Input: part model. Units: mm. Frame: model coordinates. Face numbers are marked on the shaded views. A direction names the side the tool comes from. Coordinates: 2 decimals unless noted, no trailing zeros. Write each loop counter-clockwise with the first axis right and the second up, starting at its lowest first coordinate (ties: lowest second). Pieces come first, ordered by that corner, then holes. Notation, with made-up numbers: M 6,32 L 54,32 A17 ccw 54,54 Z; hole C -8.5,24.25 d7. An arc over 180 degrees is marked long. Write each question's results on one line, items separated by ' | '. Start each with the question number.
1. Section query A-A, the plane y = 2. Output: boundary loops of the cut face in (x, z), and give its area (3 significant figures).
2. First-contact query: pin 1 (2 mm diameter, centred on x = -19, y = 25, fed in from -Z); pin 2 (0.8 mm diameter, centred on y = 27.5, z = 2, fed in from +X); pin 3 (6 mm diameter, centred on x = -16.39, y = 20, fed in from -Z); pin 4 (2 mm diameter, centred on y = 27.5, z = 4.5, fed in from -X). Flat tips, straight axial feed; report the tip coordinate or a pass-through.
3. Section query C-C, the plane y = 20. Output: boundary loops of the cut face in (x, z), and give its area (3 significant figures).
4. Pull-direction query (X, two-part tool) for the marked faces 3, 4 and 5; classes: +X half, -X half, draft (parallel to the pull), parting line (faces both ways), or undercut.
5. Ray query, probe 1 along X at (y, z) = (14.5, 5.25); probe 2 along X at (y, z) = (0, 7.75); probe 3 along Y at (x, z) = (-16.5, 6.75). Return the intervals inside material, ascending.
6. Set-up query: the marked faces 1 and 2. Return all of +Z, -Z, +X, -X, +Y, -Y with unobstructed straight access to the full face (end or side cutting, diameter ignored); none if empty.
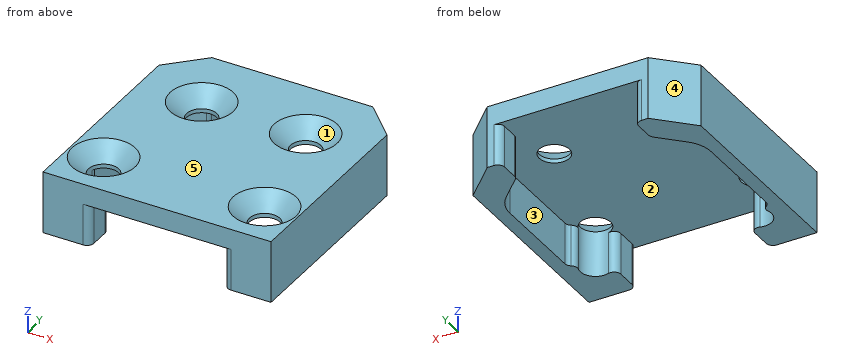
```python
from build123d import *

# Parameters (mm, degrees)
EXTRUDE1_DEPTH                                       = 9.25
CSK_FOR_M4_COUNTERSUNK_RAISED_HEAD_SCREW_D           = 4.5
CSK_FOR_M4_COUNTERSUNK_RAISED_HEAD_SCREW_CSINK_D     = 9.4
CSK_FOR_M4_COUNTERSUNK_RAISED_HEAD_SCREW_CSINK_ANGLE = 90
EXTRUDE2_DEPTH                                       = 6.2
FILLET1_R                                            = 1
FILLET2_R                                            = 1
FILLET3_R                                            = 5


with BuildPart() as part:
    # Sketch1 → Extrude1 (new body)
    with BuildSketch(Plane.XY):
        Polygon((3.357375606748374, 30), (-20.6426243932516, 30), (-25.642624393251616, 25.000000000000007), (-25.642624393251616, -4.999999999999999), (8.357375606748393, -4.999999999999999), (8.357375606748393, 25), align=None)
    extrude(amount=EXTRUDE1_DEPTH)

    # CSK for M4 Countersunk Raised Head Screw1 (through all)
    with Locations(Plane.XY.offset(9.249999999999995)):
        with Locations((-0.892624393, 20), (-16.392624393, 20), (-20.642624393, 2), (3.357375607, 2)):
            CounterSinkHole(CSK_FOR_M4_COUNTERSUNK_RAISED_HEAD_SCREW_D / 2, CSK_FOR_M4_COUNTERSUNK_RAISED_HEAD_SCREW_CSINK_D / 2, counter_sink_angle=CSK_FOR_M4_COUNTERSUNK_RAISED_HEAD_SCREW_CSINK_ANGLE)

    # Sketch6 → Extrude2 (cut)
    with BuildSketch(Plane(origin=(0, 0, 0), x_dir=(-1, 0, 0), z_dir=(0, 0, -1))):
        with BuildLine():
            Line((-1.357375606748385, -4.999999999999999), (-1.357375606748385, 1.9999999999999944))
            ThreePointArc((-1.357375606748385, 1.9999999999999944), (-1.9431620443752904, 3.4142135623730905), (-3.357375606748387, 3.9999999999999947))
            Line((-3.357375606748387, 3.9999999999999947), (-6.357375606748384, 3.9999999999999947))
            Line((-6.357375606748384, 3.9999999999999947), (-6.357375606748382, 20.999999999999996))
            Line((-6.357375606748382, 20.999999999999996), (-1.3573756067483855, 25.999999999999996))
            Line((-1.3573756067483855, 25.999999999999996), (-1.3573756067483855, 30))
            Line((-1.3573756067483855, 30), (18.642624393251616, 30))
            Line((18.642624393251616, 30), (18.642624393251616, 25.999999999999996))
            Line((18.642624393251616, 25.999999999999996), (23.642624393251612, 20.999999999999996))
            Line((23.642624393251612, 20.999999999999996), (23.642624393251612, 3.9999999999999947))
            Line((23.642624393251612, 3.9999999999999947), (20.642624393251616, 3.9999999999999947))
            ThreePointArc((20.642624393251616, 3.9999999999999947), (19.22841083087852, 3.4142135623730896), (18.642624393251616, 1.9999999999999944))
            Line((18.642624393251616, 1.9999999999999944), (18.642624393251616, -4.999999999999999))
            Line((18.642624393251616, -4.999999999999999), (-1.357375606748385, -4.999999999999999))
        make_face()
    extrude(amount=-EXTRUDE2_DEPTH, mode=Mode.SUBTRACT)

    # Fillet1
    # the kernel refuses this fillet: 1 mm, written as the material it takes off along each edge
    with BuildSketch(Plane(origin=(1.3573756067483842, -4.999999999999999, -2.5000000000000004), x_dir=(1, 0, 0), z_dir=(0, 0, 1))) as fillet1_piece_1:
        with BuildLine():
            CenterArc((FILLET1_R, FILLET1_R), FILLET1_R, 180, 90)
            Line((0, FILLET1_R), (0, 0))
            Line((0, 0), (FILLET1_R, 0))
        make_face()
    extrude(amount=8.700000000000001, mode=Mode.SUBTRACT)
    with BuildSketch(Plane(origin=(-18.642624393251616, -4.999999999999999, -2.5000000000000004), x_dir=(-1, 0, 0), z_dir=(0, 0, 1))) as fillet1_piece_2:
        with BuildLine():
            CenterArc((FILLET1_R, -FILLET1_R), FILLET1_R, 90, 90)
            Line((0, -FILLET1_R), (0, 0))
            Line((0, 0), (FILLET1_R, 0))
        make_face()
    extrude(amount=8.700000000000001, mode=Mode.SUBTRACT)
    with BuildSketch(Plane(origin=(-18.642624393251616, 30, -2.5000000000000004), x_dir=(-1, 0, 0), z_dir=(0, 0, 1))) as fillet1_piece_3:
        with BuildLine():
            CenterArc((FILLET1_R, FILLET1_R), FILLET1_R, 180, 90)
            Line((0, FILLET1_R), (0, 0))
            Line((0, 0), (FILLET1_R, 0))
        make_face()
    extrude(amount=8.700000000000001, mode=Mode.SUBTRACT)
    with BuildSketch(Plane(origin=(1.3573756067483855, 30, -2.5000000000000004), x_dir=(1, 0, 0), z_dir=(0, 0, 1))) as fillet1_piece_4:
        with BuildLine():
            CenterArc((FILLET1_R, -FILLET1_R), FILLET1_R, 90, 90)
            Line((0, -FILLET1_R), (0, 0))
            Line((0, 0), (FILLET1_R, 0))
        make_face()
    extrude(amount=8.700000000000001, mode=Mode.SUBTRACT)
    with BuildSketch(Plane(origin=(1.3573756067483855, 25.999999999999996, -1.0355339059327398), x_dir=(0, 1, 0), z_dir=(0, 0, 1))) as fillet1_piece_5:
        with BuildLine():
            CenterArc((FILLET1_R * 0.414213562373, -FILLET1_R), FILLET1_R, 90, 44.999999999999886)
            Line((-FILLET1_R * 0.292893218813, -FILLET1_R * 0.292893218813), (0, 0))
            Line((0, 0), (FILLET1_R * 0.414213562373, 0))
        make_face()
    extrude(amount=7.23553390593274, mode=Mode.SUBTRACT)
    with BuildSketch(Plane(origin=(-18.642624393251616, 25.999999999999996, -1.0355339059327398), x_dir=(0, 1, 0), z_dir=(0, 0, 1))) as fillet1_piece_6:
        with BuildLine():
            CenterArc((FILLET1_R * 0.414213562373, FILLET1_R), FILLET1_R, 225.0000000000001, 44.999999999999886)
            Line((-FILLET1_R * 0.292893218813, FILLET1_R * 0.292893218813), (0, 0))
            Line((0, 0), (FILLET1_R * 0.414213562373, 0))
        make_face()
    extrude(amount=7.23553390593274, mode=Mode.SUBTRACT)
    with BuildSketch(Plane(origin=(4.388152013404426, 3.9999999999999947, 6.2), x_dir=(0.6476614705960325, -0.7619282246415239, 0), z_dir=(0, 0, -1))) as fillet1_piece_7:
        with BuildLine():
            CenterArc((2.093085588135569, -0.924755812678291), FILLET1_R, 112.36843760662408, 102.77681294898315)
            Line((1.275390248397613, -1.5004070363987214), (0, 0))
            ThreePointArc((0, 0), (0.8562622860554598, -0.1692994214738442), (1.71252457211092, -2e-17))
        make_face()
    extrude(amount=11.123058983359915, mode=Mode.SUBTRACT)
    with BuildSketch(Plane(origin=(1.357375606748385, 0.9692235940837892, 6.2), x_dir=(0, -1, 0), z_dir=(0, 0, -1))) as fillet1_piece_8:
        with BuildLine():
            CenterArc((2.0615528132156675, -1), FILLET1_R, 90, 107.92021314405432)
            ThreePointArc((1.110066899636628, -1.3076923077697278), (0.6845392185374297, -0.5439119848812466), (0, 0))
            Line((0, 0), (2.0615528132156675, 0))
        make_face()
    extrude(amount=11.35388203303917, mode=Mode.SUBTRACT)
    with BuildSketch(Plane(origin=(-18.642624393251616, 0.9692235931073754, 6.2), x_dir=(0, -1, 0), z_dir=(0, 0, -1))) as fillet1_piece_9:
        with BuildLine():
            CenterArc((2.061552812401989, 1), FILLET1_R, 162.07978686526982, 107.92021313473018)
            ThreePointArc((1.1100668987728768, 1.3076923076148859), (0.6845392180349299, 0.543911984936301), (0, 0))
            Line((0, 0), (2.061552812401989, 0))
        make_face()
    extrude(amount=11.353882031004975, mode=Mode.SUBTRACT)
    with BuildSketch(Plane(origin=(-21.673400799404423, 3.9999999999999947, 6.2), x_dir=(-0.6476614705905301, -0.7619282246462011, 0), z_dir=(0, 0, -1))) as fillet1_piece_10:
        with BuildLine():
            CenterArc((2.0930855881723076, 0.9247558126755415), FILLET1_R, 144.8547494166881, 102.77681297627396)
            Line((1.2753902487127007, 1.5004070367913585), (0, 0))
            ThreePointArc((0, 0), (0.8562622860704877, 0.16929942148002802), (1.7125245721409794, -5e-17))
        make_face()
    extrude(amount=11.123058984617991, mode=Mode.SUBTRACT)

    # Fillet2
    fillet2_edges = [part.edges().sort_by_distance(p)[0] for p in [
        (-23.642624393251612, 3.9999999999999947, 3.1),
        (6.357375606748384, 3.9999999999999947, 3.1),
    ]]
    fillet(fillet2_edges, radius=FILLET2_R)

    # Fillet3
    fillet3_edges = [part.edges().sort_by_distance(p)[0] for p in [
        (6.357375606748382, 20.999999999999996, 3.1),
        (-23.642624393251612, 20.999999999999996, 3.1),
    ]]
    fillet(fillet3_edges, radius=FILLET3_R)


solid = part.part
```
Answer:
1) outline: M -25.64,0 L -22.89,0 L -22.89,6.8 L -25.34,9.25 L -25.64,9.25 Z; M -18.39,6.2 L 1.11,6.2 L 1.11,6.8 L -1.34,9.25 L -15.94,9.25 L -18.39,6.8 Z; M 5.61,0 L 8.36,0 L 8.36,9.25 L 8.06,9.25 L 5.61,6.8 Z | area: 98.3 mm^2
2) pin 1: z = 0 | pin 2: x = 6.26 | pin 3: z = 6.2 | pin 4: x = -24.14
3) outline: M -25.64,0 L -23.53,0 L -23.53,6.2 L -18.64,6.2 L -18.64,6.8 L -21.09,9.25 L -25.64,9.25 Z; M -14.14,6.2 L -3.14,6.2 L -3.14,6.8 L -5.59,9.25 L -11.69,9.25 L -14.14,6.8 Z; M 1.36,6.2 L 6.24,6.2 L 6.24,0 L 8.36,0 L 8.36,9.25 L 3.81,9.25 L 1.36,6.8 Z | area: 90.5 mm^2
4) face 3: undercut | face 4: -X half | face 5: draft
5) probe 1: -25.64 to -23.64, 6.36 to 8.36 | probe 2: -25.64 to -23.14, -18.14 to 0.86, 5.86 to 8.36 | probe 3: -5 to 17.75, 22.25 to 30
6) face 1: +Z | face 2: -Z
